Geometry check sheet. Reference: the model listing, model coordinates, mm. Face numbers are marked on the shaded views. Round coordinates to 2 decimals unless told otherwise and drop trailing zeros. Order: outer loops, then holes, each group sorted by start corner. A loop starts at its lowest first (then second) coordinate and runs counter-clockwise, first axis right, second up. Notation, with made-up numbers: (-28, 47.25) - (-19, 47.25) arc R30 ccw to (-19, 82.25) - close; hole circle Ø5 at (-1.75, 48). An arc over 180 degrees is marked (long way). Return JSON: item names as keys, results as strings. Group by question number.
Q1. Sectioned sample at C-C, the plane y = 8. Record the cut outline in (x, z) (3 decimals), then the cut area to 3 significant figures.
Q2. Gauge pin test, flat ends, axial feed: pin 1 Ø7.5 at (x, z) = (0, -25.4) entering from +Y (3 decimals); pin 2 Ø8.5 at (y, z) = (23.81, 0) entering from +X; pin 3 Ø10 at (y, z) = (16, -3) entering from +X. Record the tip position at first contact, or that the pin passes through.
Q3. Material ranges on line 1 along Z through (x, y) = (-7.5, 23.5); line 2 along Y through (x, z) = (4.5, 4.5) (3 decimals); line 3 along X through (y, z) = (29.5, 13.5) (3 decimals), recorded low to high.
Q4. Sectioned sample at A-A, the plane z = 0. Record the cut outline in (x, y) (3 decimals), then the cut area to 3 significant figures.
Q5. Draft check along Z on the marked faces 1, 2 and 3. Enter one of: pulls with the +Z half, pulls with the -Z half, needs draft (parallel to the pull), parting line crosses it, or undercut.
Q6. Sectioned sample at B-B, the plane x = 0. Record the cut outline in (y, z) (3 decimals), then the cut area to 3 significant figures.
Q7. Sectioned sample at D-D, the plane z = -15. Record the cut outline in (x, y) (3 decimals).
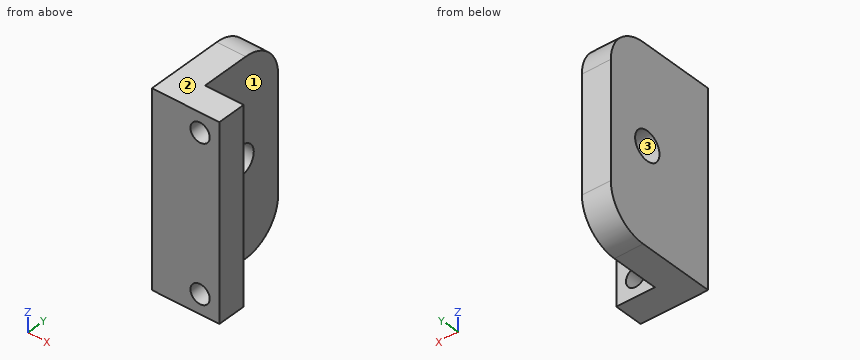
Autodesk Inventor part; units mm, degrees
ref_plane "YZ Plane" through (0, 0, 0) normal (1, 0, 0) x (0, 1, 0)
ref_plane "XZ Plane" through (0, 0, 0) normal (0, 1, 0) x (-1, 0, 0)
ref_plane "XY Plane" through (0, 0, 0) normal (0, 0, 1) x (1, 0, 0)
sketch "Sketch1" plane through (0, 0, 0) normal (0, 1, 0) x (-1, 0, 0)
  line L0 (-6.35, 31.75) -> (6.35, 31.75)
  line L1 (6.35, 31.75) -> (6.35, -31.75)
  line L2 (6.35, -31.75) -> (-6.35, -31.75)
  line L3 (-6.35, -31.75) -> (-6.35, 31.75)
  line L4 (-6.35, 31.75) -> (6.35, -31.75) construction
  line L5 (6.35, 31.75) -> (-6.35, -31.75) construction
  circle A0 centre (0, 25.4) radius 3.175
  circle A1 centre (0, -25.4) radius 3.175
  point P0 (0, 0)
  dimension "d0" = 12.7
  dimension "d1" = 63.5
  dimension "d2" = 6.35
  dimension "d3" = 6.35
  dimension "d4" = 50.8
  dimension "d5" = 6.35
extrude "Extrusion1" add sketch "Sketch1" along normal blind 9.525
sketch "Sketch2" plane through (0, 0, 0) normal (0, 1, 0) x (-1, 0, 0)
  line L0 (6.35, -31.75) -> (6.35, 31.75)
  line L1 (6.35, 31.75) -> (15.875, 31.75)
  line L2 (15.875, 31.75) -> (15.875, -31.75)
  line L3 (15.875, -31.75) -> (6.35, -31.75)
  line L4 (6.35, -31.75) -> (6.35, 31.75)
  point P0 (0, 0)
  dimension "d8" = 9.525
extrude "Extrusion2" add sketch "Sketch2" along normal blind 38.1
fillet "Fillet1" radius 12.7 2 edges at (-11.1125, 38.1, 31.75) (-11.1125, 38.1, -31.75)
sketch "Sketch3" plane through (-15.875, 0, -31.75) normal (-1, 0, 0) x (0, 0, 1)
  line L0 (50.8, 38.1) -> (12.7, 38.1)
  line L1 (31.75, 38.1) -> (31.75, 23.8125) construction
  circle A0 centre (31.75, 23.8125) radius 4.7625
  point P0 (31.75, 0)
  dimension "d12" = 14.2875
  dimension "d13" = 9.525
extrude "Extrusion3" cut sketch "Sketch3" against normal through all
equation "\"d3\" = d2"
properties part number "drum_holder" material "Aluminum 6061"
Reply:
{
 "1": {"outline": "(-15.875, -31.75) - (6.35, -31.75) - (6.35, 31.75) - (-15.875, 31.75) - close; hole circle Ø6.35 at (0, -25.4); hole circle Ø6.35 at (0, 25.4)", "area": "1,350 mm^2"},
 "2": {"pin 1": "y = 9.525", "pin 2": "through", "pin 3": "x = -6.35"},
 "3": {"line 1": "-31.75 to -4.75, 4.75 to 31.75", "line 2": "0 to 9.525", "line 3": "-15.875 to -6.35"},
 "4": {"outline": "(-15.875, 0) - (6.35, 0) - (6.35, 9.525) - (-6.35, 9.525) - (-6.35, 19.05) - (-15.875, 19.05) - close; (-15.875, 28.575) - (-6.35, 28.575) - (-6.35, 38.1) - (-15.875, 38.1) - close", "area": "393 mm^2"},
 "5": {"face 1": "needs draft", "face 2": "pulls with the +Z half", "face 3": "undercut"},
 "6": {"outline": "(0, -31.75) - (9.525, -31.75) - (9.525, -28.575) - (0, -28.575) - close; (0, -22.225) - (9.525, -22.225) - (9.525, 22.225) - (0, 22.225) - close; (0, 28.575) - (9.525, 28.575) - (9.525, 31.75) - (0, 31.75) - close", "area": "484 mm^2"},
 "7": {"outline": "(-15.875, 0) - (6.35, 0) - (6.35, 9.525) - (-6.35, 9.525) - (-6.35, 38.1) - (-15.875, 38.1) - close"}
}
